Geometry check sheet. Reference: the model listing, model coordinates, mm. Give positions to 0.01 mm unless a question says otherwise; leave off trailing zeros. Order: outer loops, then holes, each group sorted by start corner. A loop starts at its lowest first (then second) coordinate and runs counter-clockwise, first axis right, second up.
from build123d import *

# Parameters (mm, degrees)
BOSS_EXTRUDE1_DEPTH = 6.35
SKETCH3_R           = 2.499999953
CUT_EXTRUDE1_DEPTH  = 6.35
LPATTERN1_COUNT     = 2
LPATTERN1_PITCH     = 139.7


with BuildPart() as part:
    # Sketch1 → Boss-Extrude1 (new body)
    with BuildSketch(Plane(origin=(0, 0, 0), x_dir=(1, 0, 0), z_dir=(0, 1, 0))):
        with BuildLine():
            Line((0, 12.7), (139.7, 12.7))
            ThreePointArc((139.7, 12.7), (152.4, 0), (139.7, -12.7))
            Line((139.7, -12.7), (0, -12.7))
            ThreePointArc((0, -12.7), (-12.7, 0), (0, 12.7))
        make_face()
    extrude(amount=BOSS_EXTRUDE1_DEPTH)

    # Sketch3 → Cut-Extrude1 (cut)
    with BuildSketch(Plane(origin=(0, 6.35, 0), x_dir=(1, 0, 0), z_dir=(0, 1, 0))):
        with Locations(Location((0, 0, 0), (0, 0, 270))):
            Circle(SKETCH3_R)
    cut_extrude1 = extrude(amount=-CUT_EXTRUDE1_DEPTH, mode=Mode.SUBTRACT)

    # LPattern1: Cut-Extrude1 ×2
    with Locations(*[(i * LPATTERN1_PITCH, 0, 0) for i in range(1, LPATTERN1_COUNT)]):
        add(cut_extrude1, mode=Mode.SUBTRACT)


solid = part.part
Item 1: Gauge pin test, flat ends, axial feed: pin 1 (5 mm diameter, centred on x = 25, z = -2, fed in from -Y); pin 2 (1.5 mm diameter, centred on y = 2, z = -4, fed in from +X). Record the tip position at first contact, or that the pin passes through.
Reported:
pin 1: stops at y = 0
pin 2: stops at x = 151.98
Item 2: Draft check along X on faces 1 (the cylindrical face through (152.397, 3.131, -0.279)), 2 (the cylindrical face through (137.26, 3.22, -0.54)), 3 (the flat face through (71, 0, 0)). Enter one of: released by +X, released by -X, zero draft, split by the parting line, or undercut.
Reported:
face 1: released by +X
face 2: undercut
face 3: zero draft
Item 3: Sectioned sample at A-A (z = 0). Enter the section's corners in (x, y).
Reported:
outline: (-12.7, 0) - (-2.5, 0) - (-2.5, 6.35) - (-12.7, 6.35) - close; (2.5, 0) - (137.2, 0) - (137.2, 6.35) - (2.5, 6.35) - close; (142.2, 0) - (152.4, 0) - (152.4, 6.35) - (142.2, 6.35) - close
Item 4: Scan lines: L1, parallel to X at y = 3.75, z = 0; L2, parallel to Z at x = 0, y = 5; L3, parallel to X at y = 2.5, z = -1. Record each from-to range of solid material in increasing order.
Reported:
L1: x = -12.7 to -2.5, 2.5 to 137.2, 142.2 to 152.4
L2: z = -12.7 to -2.5, 2.5 to 12.7
L3: x = -12.66 to -2.29, 2.29 to 137.41, 141.99 to 152.36
Item 5: Sectioned sample at B-B (y = 3.25). Enter the section's corners in (x, z).
Reported:
outline: (0, -12.7) - (139.7, -12.7) arc R12.7 ccw to (139.7, 12.7) - (0, 12.7) arc R12.7 ccw to start; hole circle Ø5 at (0, 0); hole circle Ø5 at (139.7, 0)
Item 6: Sectioned sample at C-C (z = -7.25). Enter the section's corners in (x, y), and give its area (3 significant figures).
Reported:
outline: (-10.43, 0) - (150.13, 0) - (150.13, 6.35) - (-10.43, 6.35) - close
area: 1,020 mm2
